The drawing under review shows one solid part. Ordinate dimensions are in mm from its lowest x, y, z. A direction names the side the tool comes from. Round coordinates to 2 decimals unless told otherwise and drop trailing zeros. Write each loop counter-clockwise with the first axis right and the second up, starting at its lowest first coordinate (ties: lowest second). Pieces come first, ordered by that corner, then holes. Notation, with made-up numbers: M 74,12 L 91,12 A18 ccw 91,28 Z; hole C -15,-37.75 d6. An arc over 180 degrees is marked long. Write item = value, one per line. Start each with the question number.
Item 1: Tool access review of the marked faces 1 and 2: name each direction out of +Z, -Z, +X, -X, +Y, -Y from which nothing blocks a thin tool from reaching the whole face with its end or side.
Item 2: Take a section at A-A, the plane z = 74.5. Give the boundary of the cut face in (x, y), plus the area to 3 significant figures.
Item 3: To check wall thickness, follow line 1 along Z through (x, y) = (351, 12); line 2 along Y through (x, z) = (154, 61); line 3 along X through (y, z) = (26.5, 339). State the ranges of each line that lie inside material, in increasing order.
Item 4: Take a section at C-C, the plane y = 21. Give the boundary of the cut face in (x, z), plus the area to 3 significant figures.
Item 5: The part is to be moulded in two halves that separate along Y. For the marked faces 3 and 4, say which applies: +Y half, -Y half, draft (parallel to the pull), parting line (faces both ways), or undercut.
Item 6: Take a section at B-B, the plane x = 183.5. Give the boundary of the cut face in (y, z).
Item 7: For pin 1 Ø6.5 at (y, z) = (12.7, 317.5) entering from -X; pin 2 Ø3 at (y, z) = (17, 136.5) entering from -X; pin 3 Ø12 at (x, z) = (312.5, 101) entering from -Y (1 decimal); pin 4 Ø1.9 at (x, z) = (346, 225.5) entering from -Y, all flat-tipped, find the tip position at first contact; note any pin that passes through.
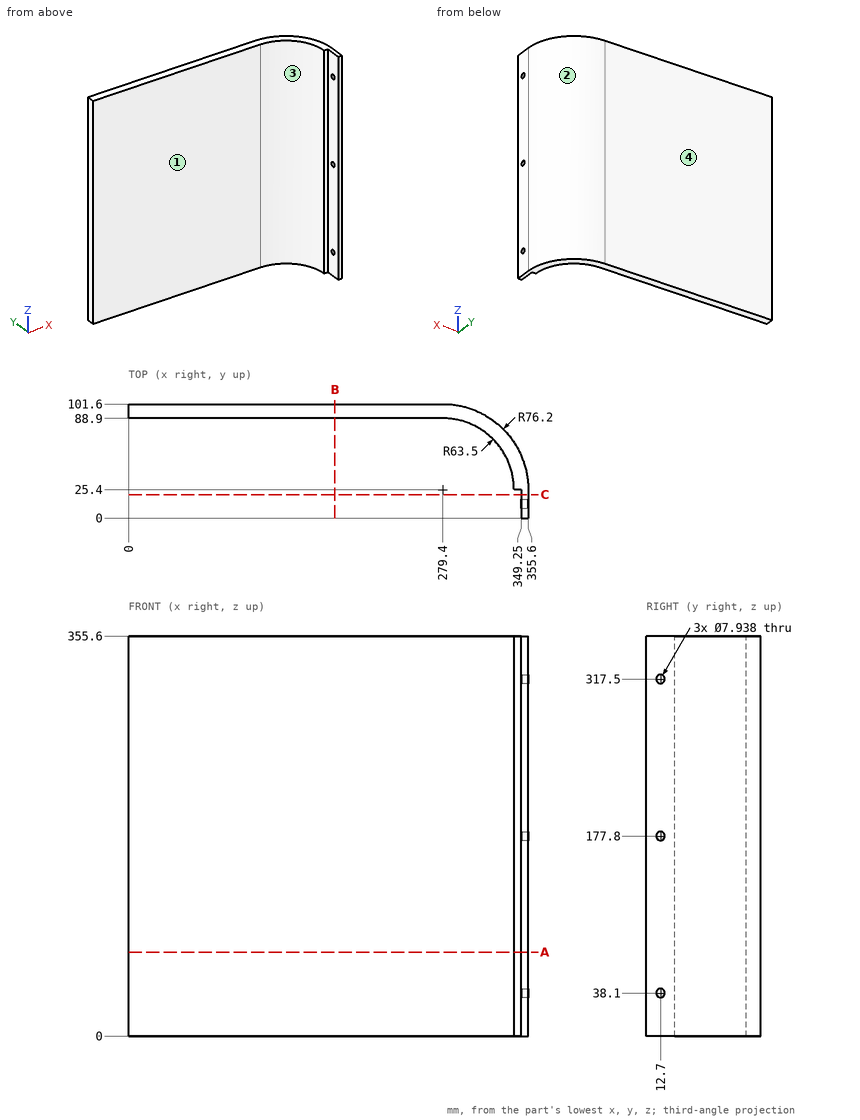
Response values:
q1.face_1 = +Z, -Z, -X, -Y
q1.face_2 = +Z, -Z, +X, +Y
q2.outline = M 0,88.9 L 279.4,88.9 A63.5 cw 342.9,25.4 L 349.25,25.4 L 349.25,0 L 355.6,0 L 355.6,25.4 A76.2 ccw 279.4,101.6 L 0,101.6 Z
q2.area = 5,100 mm2
q3.line_1 = 0 to 34.19, 42.01 to 173.89, 181.71 to 313.59, 321.41 to 355.6
q3.line_2 = 88.9 to 101.6
q3.line_3 = 342.89 to 355.59
q4.outline = M 349.25,0 L 355.6,0 L 355.6,355.6 L 349.25,355.6 Z
q4.area = 2,260 mm2
q5.face_3 = -Y half
q5.face_4 = +Y half
q6.outline = M 88.9,0 L 101.6,0 L 101.6,355.6 L 88.9,355.6 Z
q7.pin_1 = through
q7.pin_2 = 349.25
q7.pin_3 = 75.4
q7.pin_4 = 25.4
